Read the model definition and answer for the solid it produces. Units are mm, in the model's axes. A direction names the side the tool comes from. Coordinates: 2 decimals unless noted, no trailing zeros. Write each loop counter-clockwise with the first axis right and the second up, starting at its lowest first coordinate (ties: lowest second). Pieces come first, ordered by that corner, then holes. Notation, with made-up numbers: (61, -9.5) -> (113, -9.5) arc R12 ccw to (113, 4.5) -> close; hole circle Ø3 at (-25.75, 56.25). An arc over 180 degrees is marked (long way). Return JSON: item names as keys, results as strings.
from build123d import *

# Parameters (mm, degrees)
F0_R     = 40
F0_R_2   = 15.05
F1_DEPTH = 5
F0_R_3   = 8.45
F2_DEPTH = 4
F0_R_4   = 7.5
F3_DEPTH = 5
F0_R_5   = 4
F4_DEPTH = 13
F5_DEPTH = 20
F6_SIZE2 = 2
F6_SIZE  = 2


with BuildPart() as f1:
    # F0 (on Top) → F1 (new body)
    with BuildSketch(Plane.XY):
        Circle(F0_R)
        with BuildLine():
            ThreePointArc((-11.9611435045, -30.6375331929), (-19.0718793869, -33.0334640939), (-20.5523103021, -25.6774207297))
            Line((-20.5523103021, -25.6774207297), (-13.4086800794, -16.2803577113))
            ThreePointArc((-13.4086800794, -16.2803577113), (-8.8723784387, -15.3674102398), (-7.394863321, -19.7524364356))
            Line((-7.394863321, -19.7524364356), (-11.9611435045, -30.6375331929))
        make_face(mode=Mode.SUBTRACT)
        with BuildLine():
            ThreePointArc((4.9601124633, -32.5134538066), (0, -38.1437587738), (-4.9601124633, -32.5134538066))
            Line((-4.9601124633, -32.5134538066), (-3.4720787243, -20.8035434004))
            ThreePointArc((-3.4720787243, -20.8035434004), (0, -17.7447568774), (3.4720787243, -20.8035434004))
            Line((3.4720787243, -20.8035434004), (4.9601124633, -32.5134538066))
        make_face(mode=Mode.SUBTRACT)
        with BuildLine():
            ThreePointArc((-25.6774207297, -20.5523103021), (-33.0334640939, -19.0718793869), (-30.6375331929, -11.9611435045))
            Line((-30.6375331929, -11.9611435045), (-19.7524364356, -7.394863321))
            ThreePointArc((-19.7524364356, -7.394863321), (-15.3674102398, -8.8723784387), (-16.2803577113, -13.4086800794))
            Line((-16.2803577113, -13.4086800794), (-25.6774207297, -20.5523103021))
        make_face(mode=Mode.SUBTRACT)
        with BuildLine():
            ThreePointArc((20.5523103021, -25.6774207297), (19.0718793869, -33.0334640939), (11.9611435045, -30.6375331929))
            Line((11.9611435045, -30.6375331929), (7.394863321, -19.7524364356))
            ThreePointArc((7.394863321, -19.7524364356), (8.8723784387, -15.3674102398), (13.4086800794, -16.2803577113))
            Line((13.4086800794, -16.2803577113), (20.5523103021, -25.6774207297))
        make_face(mode=Mode.SUBTRACT)
        with BuildLine():
            ThreePointArc((30.6375331929, -11.9611435045), (33.0334640939, -19.0718793869), (25.6774207297, -20.5523103021))
            Line((25.6774207297, -20.5523103021), (16.2803577113, -13.4086800794))
            ThreePointArc((16.2803577113, -13.4086800794), (15.3674102398, -8.8723784387), (19.7524364356, -7.394863321))
            Line((19.7524364356, -7.394863321), (30.6375331929, -11.9611435045))
        make_face(mode=Mode.SUBTRACT)
        with BuildLine():
            ThreePointArc((32.5134538066, 4.9601124633), (38.1437587738, 0), (32.5134538066, -4.9601124633))
            Line((32.5134538066, -4.9601124633), (20.8035434004, -3.4720787243))
            ThreePointArc((20.8035434004, -3.4720787243), (17.7447568774, 0), (20.8035434004, 3.4720787243))
            Line((20.8035434004, 3.4720787243), (32.5134538066, 4.9601124633))
        make_face(mode=Mode.SUBTRACT)
        with BuildLine():
            ThreePointArc((-32.5134538066, -4.9601124633), (-38.1437587738, 0), (-32.5134538066, 4.9601124633))
            Line((-32.5134538066, 4.9601124633), (-20.8035434004, 3.4720787243))
            ThreePointArc((-20.8035434004, 3.4720787243), (-17.7447568774, 0), (-20.8035434004, -3.4720787243))
            Line((-20.8035434004, -3.4720787243), (-32.5134538066, -4.9601124633))
        make_face(mode=Mode.SUBTRACT)
        with BuildLine():
            ThreePointArc((-30.6375331929, 11.9611435045), (-33.0334640939, 19.0718793869), (-25.6774207297, 20.5523103021))
            Line((-25.6774207297, 20.5523103021), (-16.2803577113, 13.4086800794))
            ThreePointArc((-16.2803577113, 13.4086800794), (-15.3674102398, 8.8723784387), (-19.7524364356, 7.394863321))
            Line((-19.7524364356, 7.394863321), (-30.6375331929, 11.9611435045))
        make_face(mode=Mode.SUBTRACT)
        with BuildLine():
            ThreePointArc((-20.5523103021, 25.6774207297), (-19.0718793869, 33.0334640939), (-11.9611435045, 30.6375331929))
            Line((-11.9611435045, 30.6375331929), (-7.394863321, 19.7524364356))
            ThreePointArc((-7.394863321, 19.7524364356), (-8.8723784387, 15.3674102398), (-13.4086800794, 16.2803577113))
            Line((-13.4086800794, 16.2803577113), (-20.5523103021, 25.6774207297))
        make_face(mode=Mode.SUBTRACT)
        Circle(F0_R_2, mode=Mode.SUBTRACT)
        with BuildLine():
            ThreePointArc((25.6774207297, 20.5523103021), (33.0334640939, 19.0718793869), (30.6375331929, 11.9611435045))
            Line((30.6375331929, 11.9611435045), (19.7524364356, 7.394863321))
            ThreePointArc((19.7524364356, 7.394863321), (15.3674102398, 8.8723784387), (16.2803577113, 13.4086800794))
            Line((16.2803577113, 13.4086800794), (25.6774207297, 20.5523103021))
        make_face(mode=Mode.SUBTRACT)
        with BuildLine():
            ThreePointArc((3.4720787243, 20.8035434004), (0, 17.7447568774), (-3.4720787243, 20.8035434004))
            Line((-3.4720787243, 20.8035434004), (-4.9601124633, 32.5134538066))
            ThreePointArc((-4.9601124633, 32.5134538066), (0, 38.1437587738), (4.9601124633, 32.5134538066))
            Line((4.9601124633, 32.5134538066), (3.4720787243, 20.8035434004))
        make_face(mode=Mode.SUBTRACT)
        with BuildLine():
            ThreePointArc((11.9611435045, 30.6375331929), (19.0718793869, 33.0334640939), (20.5523103021, 25.6774207297))
            Line((20.5523103021, 25.6774207297), (13.4086800794, 16.2803577113))
            ThreePointArc((13.4086800794, 16.2803577113), (8.8723784387, 15.3674102398), (7.394863321, 19.7524364356))
            Line((7.394863321, 19.7524364356), (11.9611435045, 30.6375331929))
        make_face(mode=Mode.SUBTRACT)
    extrude(amount=F1_DEPTH)

    # F0 (on Top) → F2 (join)
    with BuildSketch(Plane.XY):
        Circle(F0_R_2)
        Circle(F0_R_3, mode=Mode.SUBTRACT)
    extrude(amount=F2_DEPTH)

    # F0 (on Top) → F3 (join)
    with BuildSketch(Plane.XY):
        Circle(F0_R_3)
        Circle(F0_R_4, mode=Mode.SUBTRACT)
    extrude(amount=F3_DEPTH)

    # F0 (on Top) → F4 (join)
    with BuildSketch(Plane.XY):
        Circle(F0_R_4)
        Circle(F0_R_5, mode=Mode.SUBTRACT)
    extrude(amount=F4_DEPTH)

    # F0 (on Top) → F5 (join)
    with BuildSketch(Plane.XY):
        Circle(F0_R_5)
    extrude(amount=F5_DEPTH)

    # F6
    f6_edges = [f1.edges().sort_by_distance(p)[0] for p in [
        (-4, 0, 20),
    ]]
    chamfer(f6_edges, length=F6_SIZE, length2=F6_SIZE2)


solid = f1.part
1. For a pull along Y with two mould halves and no side action, classify faces 3 (the face through (8.06, 2.54, 4.49)), 4 (the face through (-7.493, 0.33, 8.944)), 5 (the face through (3, -3, 13)) as +Y half, -Y half, draft (parallel to the pull), parting line (faces both ways), or undercut.
Taken from the geometry:
{"face 3": "undercut", "face 4": "parting line", "face 5": "draft"}
2. Consider L1, parallel to X at y = -20.5, z = 1.5; L2, parallel to Z at x = 36, y = 7; L3, parallel to X at y = -2, z = 15.5. Determine where each line is inside the solid, lowest interval first.
Taken from the geometry:
{"L1": "x = -34.35 to -31.8, -25.61 to -16.62, -7.71 to -3.42, 3.42 to 7.71, 16.62 to 25.61, 31.8 to 34.35", "L2": "z = 0 to 5", "L3": "x = -3.46 to 3.46"}
3. The part is cut by section A-A (x = 0). Count the separate pieces of the cut face and the enclosed holes in it, then the cut area to 3 significant figures.
Taken from the geometry:
{"separate pieces": "3", "enclosed holes": "0", "area": "355 mm2"}
4. The part is cut by section D-D (z = 6.5). Determine the outline of the cut face in (x, y).
Taken from the geometry:
{"outline": "circle Ø15 at (0, 0)"}
5. A tool of negligible diameter and unlimited length cuts with its end or side. For faces 1 (the face through (-5, -6, 5)), 2 (the face through (-17.031, -21.045, 2.465)), from which of +Z, -Z, +X, -X, +Y, -Y can it reach the whole face along a straight path? Write none if from no direction.
Taken from the geometry:
{"face 1": "+Z", "face 2": "+Z, -Z"}
6. The part is cut by section B-B (y = -23.5). Determine the outline of the cut face in (x, z), then the cut area to 3 significant figures.
Taken from the geometry:
{"outline": "(-32.37, 0) -> (-18.9, 0) -> (-18.9, 5) -> (-32.37, 5) -> close; (-8.97, 0) -> (-3.81, 0) -> (-3.81, 5) -> (-8.97, 5) -> close; (3.81, 0) -> (8.97, 0) -> (8.97, 5) -> (3.81, 5) -> close; (18.9, 0) -> (32.37, 0) -> (32.37, 5) -> (18.9, 5) -> close", "area": "186 mm2"}
7. Flat-ended cylindrical pins translate along their axes: pin 1 Ø6 at (x, y) = (-28.7, -16.57) entering from +Z; pin 2 Ø11.5 at (x, y) = (-33.14, 0) entering from +Z; pin 3 Ø12 at (x, y) = (-9, -15) entering from -Z. Find the tip coordinate at first contact, or state that the pin passes through.
Taken from the geometry:
{"pin 1": "passes through", "pin 2": "stops at z = 5", "pin 3": "stops at z = 0"}
